Could you check a few things on this model? Use its own coordinates, in mm. A direction names the side the tool comes from. Give positions to 0.01 mm unless a question says otherwise; leave off trailing zeros. Write each loop counter-clockwise with the first axis right and the second up, starting at its lowest first coordinate (ties: lowest second). Pieces come first, ordered by that corner, then holes. Notation, with made-up numbers: M 39.25,-18 L 83.25,-18 A9 cw 83.25,-11 Z; hole C -37,80 d3. An arc over 180 degrees is marked long. One line per item, written item: value.
```python
from build123d import *
from build123d.topology import SkipClean

# Parameters (mm, degrees)
BOSS_EXTRUDE1_DEPTH     = 3.25
BOSS_EXTRUDE2_START     = 2.5
SKETCH2_R               = 3.5
BOSS_EXTRUDE2_DEPTH     = 2.5
SKETCH3_R               = 5
BOSS_EXTRUDE3_DEPTH     = 0.5
BOSS_EXTRUDE4_DEPTH     = 8.25
SKETCH6_W               = 0.5
SKETCH6_H               = 0.45
CUT_EXTRUDE1_DEPTH      = 8.25
LPATTERN1_COUNT         = 4
LPATTERN1_PITCH         = 0.9
MIRROR1_COPY_1_SKETCH_W = 0.5
MIRROR1_COPY_1_SKETCH_H = 0.45
MIRROR1_COPY_1_DEPTH    = 8.25
MIRROR1_COPY_2_SKETCH_W = 0.5
MIRROR1_COPY_2_SKETCH_H = 0.45
MIRROR1_COPY_2_DEPTH    = 8.25
MIRROR1_COPY_3_SKETCH_W = 0.5
MIRROR1_COPY_3_SKETCH_H = 0.45
MIRROR1_COPY_3_DEPTH    = 8.25
SKETCH7_R               = 3
CUT_EXTRUDE2_DEPTH      = 9
SKETCH7_4_R             = 0.75
CUT_EXTRUDE3_DEPTH      = 14.107726729
CUT_EXTRUDE4_REACH      = 15.108
SKETCH7_5_R             = 0.375


with BuildPart() as part:
    # Sketch1 → Boss-Extrude1 (new, symmetric)
    with BuildSketch(Plane.XY):
        with BuildLine():
            Line((-6, -6.75), (6, -6.75))
            Line((6, -6.75), (3.312648335, 1.129761483))
            ThreePointArc((3.312648335, 1.129761483), (0, 3.5), (-3.312648335, 1.129761483))
            Line((-3.312648335, 1.129761483), (-6, -6.75))
        make_face()
    extrude(amount=BOSS_EXTRUDE1_DEPTH, both=True)

    # Sketch2 → Boss-Extrude2 (add)
    with SkipClean():  # the faces are left unmerged after this step: merging them gives an invalid solid
        with BuildSketch(Plane.XY.offset(3.25).offset(BOSS_EXTRUDE2_START)):
            with Locations(Location((0, 0, 0), (0, 0, 161.168324383))):
                Circle(SKETCH2_R)
        extrude(amount=-BOSS_EXTRUDE2_DEPTH)

    # Sketch3 → Boss-Extrude3 (add)
    with BuildSketch(Plane.XY.offset(5.75)):
        Circle(SKETCH3_R)
    extrude(amount=BOSS_EXTRUDE3_DEPTH)

    # Sketch5 → Boss-Extrude4 (add)
    with SkipClean():  # the faces are left unmerged after this step: merging them gives an invalid solid
        with BuildSketch(Plane(origin=(0, 0, 5.75), x_dir=(-1, 0, 0), z_dir=(0, 0, -1))):
            with BuildLine():
                Line((3, 6), (-3, 6))
                Line((-3, 6), (-3, 1.802775638))
                ThreePointArc((-3, 1.802775638), (0, 3.5), (3, 1.802775638))
                Line((3, 1.802775638), (3, 6))
            make_face()
        extrude(amount=BOSS_EXTRUDE4_DEPTH)

    # Sketch6 → Cut-Extrude1 (cut)
    with SkipClean():  # the faces are left unmerged after this step: merging them gives an invalid solid
        with BuildSketch(Plane(origin=(0, 0, -2.5), x_dir=(-1, 0, 0), z_dir=(0, 0, -1))):
            with Locations((-2.75, 5.325)):
                Rectangle(SKETCH6_W, SKETCH6_H)
        cut_extrude1 = extrude(amount=-CUT_EXTRUDE1_DEPTH, mode=Mode.SUBTRACT)

    # LPattern1: Cut-Extrude1 ×4
    with SkipClean():  # the faces are left unmerged after this step: merging them gives an invalid solid
        with Locations(*[(0, -i * LPATTERN1_PITCH, 0) for i in range(1, LPATTERN1_COUNT)]):
            add(cut_extrude1, mode=Mode.SUBTRACT)

    # Mirror1: Cut-Extrude1 across plane
    with SkipClean():  # the faces are left unmerged after this step: merging them gives an invalid solid
        add(cut_extrude1.mirror(Plane(origin=(0, 0, 0), x_dir=(0, 0, 1), z_dir=(1, 0, 0))), mode=Mode.SUBTRACT)

    # Mirror1 copy 1 sketch → Mirror1 copy 1 (cut)
    with SkipClean():  # the faces are left unmerged after this step: merging them gives an invalid solid
        with BuildSketch(Plane(origin=(0, -0.9, -2.5), x_dir=(1, 0, 0), z_dir=(0, 0, -1))):
            with Locations((-2.75, -5.325)):
                Rectangle(MIRROR1_COPY_1_SKETCH_W, MIRROR1_COPY_1_SKETCH_H)
        extrude(amount=-MIRROR1_COPY_1_DEPTH, mode=Mode.SUBTRACT)

    # Mirror1 copy 2 sketch → Mirror1 copy 2 (cut)
    with SkipClean():  # the faces are left unmerged after this step: merging them gives an invalid solid
        with BuildSketch(Plane(origin=(0, -1.8, -2.5), x_dir=(1, 0, 0), z_dir=(0, 0, -1))):
            with Locations((-2.75, -5.325)):
                Rectangle(MIRROR1_COPY_2_SKETCH_W, MIRROR1_COPY_2_SKETCH_H)
        extrude(amount=-MIRROR1_COPY_2_DEPTH, mode=Mode.SUBTRACT)

    # Mirror1 copy 3 sketch → Mirror1 copy 3 (cut)
    with SkipClean():  # the faces are left unmerged after this step: merging them gives an invalid solid
        with BuildSketch(Plane(origin=(0, -2.7, -2.5), x_dir=(1, 0, 0), z_dir=(0, 0, -1))):
            with Locations((-2.75, -5.325)):
                Rectangle(MIRROR1_COPY_3_SKETCH_W, MIRROR1_COPY_3_SKETCH_H)
        extrude(amount=-MIRROR1_COPY_3_DEPTH, mode=Mode.SUBTRACT)

    # Sketch7 → Cut-Extrude2 (cut)
    with SkipClean():  # the faces are left unmerged after this step: merging them gives an invalid solid
        with BuildSketch(Plane.XY.offset(6.25)):
            Circle(SKETCH7_R)
        extrude(amount=-CUT_EXTRUDE2_DEPTH, mode=Mode.SUBTRACT)

    # Sketch7_4 → Cut-Extrude3 (cut, through all)
    with SkipClean():  # the faces are left unmerged after this step: merging them gives an invalid solid
        with BuildSketch(Plane.XY.offset(6.25)):
            Circle(SKETCH7_4_R)
        extrude(amount=-CUT_EXTRUDE3_DEPTH, mode=Mode.SUBTRACT)

    # Sketch7_5 → Cut-Extrude4 (cut, up to next)
    with BuildSketch(Plane.XY.offset(6.25), mode=Mode.PRIVATE) as cut_extrude4_sk1:
        with Locations((0, -4.25)):
            Circle(SKETCH7_5_R)
    cut_extrude4_tool1 = extrude(cut_extrude4_sk1.sketch, amount=-CUT_EXTRUDE4_REACH, mode=Mode.PRIVATE) & part.part
    # Sketch7_5 → Cut-Extrude4 (cut, up to next)
    with BuildSketch(Plane.XY.offset(6.25), mode=Mode.PRIVATE) as cut_extrude4_sk2:
        with Locations((-3.680607966, 2.125)):
            Circle(SKETCH7_5_R)
    cut_extrude4_tool2 = extrude(cut_extrude4_sk2.sketch, amount=-CUT_EXTRUDE4_REACH, mode=Mode.PRIVATE) & part.part
    # Sketch7_5 → Cut-Extrude4 (cut, up to next)
    with BuildSketch(Plane.XY.offset(6.25), mode=Mode.PRIVATE) as cut_extrude4_sk3:
        with Locations((3.680607966, 2.125)):
            Circle(SKETCH7_5_R)
    cut_extrude4_tool3 = extrude(cut_extrude4_sk3.sketch, amount=-CUT_EXTRUDE4_REACH, mode=Mode.PRIVATE) & part.part
    add(cut_extrude4_tool1.solids().sort_by_distance((0, -4.25, 6.25))[0], mode=Mode.SUBTRACT)
    add(cut_extrude4_tool2.solids().sort_by_distance((-3.680608, 2.125, 6.25))[0], mode=Mode.SUBTRACT)
    add(cut_extrude4_tool3.solids().sort_by_distance((3.680608, 2.125, 6.25))[0], mode=Mode.SUBTRACT)


solid = part.part
```
1) I'm going to push flat-ended pins straight in: pin 1 (3 mm diameter, centred on y = 2.5, z = 0.5, fed in from -X); pin 2 (3 mm diameter, centred on x = -0.5, y = -1, fed in from +Z); pin 3 (1.5 mm diameter, centred on y = 3, z = 0.5, fed in from +X). Where does each tip first touch, or does it pass through?
Outcome:
pin 1: stops at x = -3.36
pin 2: stops at z = -2.75
pin 3: stops at x = 3
2) If we section it at B-B, the plane x = 0: Write out the boundary of the cut face in (y, z) (3 decimals), then the cut area to 3 significant figures.
Outcome:
outline: M -6.75,-3.25 L -0.75,-3.25 L -0.75,-2.75 L -3,-2.75 L -3,6.25 L -3.875,6.25 L -3.875,5.75 L -3.5,5.75 L -3.5,3.25 L -6.75,3.25 Z; M -5,5.75 L -4.625,5.75 L -4.625,6.25 L -5,6.25 Z; M 0.75,-3.25 L 3.5,-3.25 L 3.5,-2.5 L 6,-2.5 L 6,5.75 L 5,5.75 L 5,6.25 L 3,6.25 L 3,-2.75 L 0.75,-2.75 Z
area: 54.6 mm^2
3) We'd pull the mould along X, two halves only. Please class faces 6 (the face through (4.675, -2.865, 0.046)), 7 (the face through (0, -5, 3.25)), 8 (the face through (-3, 0, 2)): pulls with the +X half, pulls with the -X half, needs draft (parallel to the pull), parting line crosses it, or undercut.
Outcome:
face 6: pulls with the +X half
face 7: needs draft
face 8: undercut
4) If we section it at D-D, the plane x = -4.5: Write out the boundary of the cut face in (y, z).
Outcome:
outline: M -6.75,-3.25 L -2.35,-3.25 L -2.35,3.25 L -6.75,3.25 Z; M -2.18,5.75 L 2.18,5.75 L 2.18,6.25 L -2.18,6.25 Z
5) If we section it at C-C, the plane y = -4.25: Write out the boundary of the cut face in (x, z) (3 decimals).
Outcome:
outline: M -5.147,-3.25 L 5.147,-3.25 L 5.147,3.25 L -5.147,3.25 Z; M -2.634,5.75 L -0.375,5.75 L -0.375,6.25 L -2.634,6.25 Z; M 0.375,5.75 L 2.634,5.75 L 2.634,6.25 L 0.375,6.25 Z
6) Please list where these lines run through material, in increasing order: L1, parallel to Y at x = -0.25, z = 6; L2, parallel to Y at x = 0, z = 6.15 (3 decimals); L3, parallel to Z at x = 0.5, y = 5.5. Write a range as from..to.
Outcome:
L1: y = -4.99..-4.53, -3.97..-2.99, 2.99..4.99
L2: y = -5..-4.625, -3.875..-3, 3..5
L3: z = -2.5..5.75
7) On a 3-axis mill with a long thin cutter (end or side, diameter ignored), from which of +Z, -Z, +X, -X, +Y, -Y can I reach the whole of each face in a straight line? I mean faces 1 (the face through (0, 5.4, 5.75)), 2 (the face through (3.3, 0.1, 6.25)), 3 (the face through (0, -3, -3.25)), 4 (the face through (-4.638, -2.755, 0.046)), 5 (the face through (1, -1, -2.75)). Say none if no direction works.
Outcome:
face 1: +Z, +Y
face 2: +Z, +X, -X, +Y, -Y
face 3: -Z, +X, -X, +Y, -Y
face 4: -Z, -X, +Y
face 5: +Z
8) If we section it at A-A, the plane y = 0: Write out the boundary of the cut face in (x, z).
Outcome:
outline: M -5,5.75 L -3.5,5.75 L -3.5,3.25 L -3.7,3.25 L -3.7,-3.25 L -0.75,-3.25 L -0.75,-2.75 L -3,-2.75 L -3,6.25 L -5,6.25 Z; M 0.75,-3.25 L 3.7,-3.25 L 3.7,3.25 L 3.5,3.25 L 3.5,5.75 L 5,5.75 L 5,6.25 L 3,6.25 L 3,-2.75 L 0.75,-2.75 Z
